from build123d import *

# Parameters (mm, degrees)
SKETCH2_W           = 25.4
SKETCH2_H           = 25.4
BOSS_EXTRUDE1_DEPTH = 279.4
SKETCH4_W           = 19.05
SKETCH4_H           = 10.16
CUT_EXTRUDE1_DEPTH  = 280.9766776
SKETCH5_R           = 3.2639
CUT_EXTRUDE2_DEPTH  = 281.839473721
SKETCH6_R           = 3.2639
CUT_EXTRUDE3_DEPTH  = 281.839473721


with BuildPart() as part:
    # Sketch2 → Boss-Extrude1 (new body)
    with BuildSketch(Plane.XY):
        Rectangle(SKETCH2_W, SKETCH2_H)
    extrude(amount=BOSS_EXTRUDE1_DEPTH)

    # Sketch4 → Cut-Extrude1 (cut, through all)
    with BuildSketch(Plane.XY):
        Rectangle(SKETCH4_W, SKETCH4_H)
    extrude(amount=CUT_EXTRUDE1_DEPTH, mode=Mode.SUBTRACT)

    # Sketch5 → Cut-Extrude2 (cut, through all)
    with BuildSketch(Plane(origin=(0, 12.7, 0), x_dir=(1, 0, 0), z_dir=(0, 1, 0))):
        with Locations(Location((0, -15.24, 0), (0, 0, 270))):
            Circle(SKETCH5_R)
    extrude(amount=-CUT_EXTRUDE2_DEPTH, mode=Mode.SUBTRACT)

    # Sketch6 → Cut-Extrude3 (cut, through all)
    with BuildSketch(Plane(origin=(0, 12.7, 0), x_dir=(1, 0, 0), z_dir=(0, 1, 0))):
        with Locations(Location((0, -228.6, 0), (0, 0, 270))):
            Circle(SKETCH6_R)
    extrude(amount=-CUT_EXTRUDE3_DEPTH, mode=Mode.SUBTRACT)


solid = part.part
Source: CAD feature listing. Evaluate the final solid. Frame: model axes, mm. A direction names the side the tool comes from. Give positions to 0.01 mm unless a question says otherwise; leave off trailing zeros. Order: outer loops, then holes, each group sorted by start corner. A loop starts at its lowest first (then second) coordinate and runs counter-clockwise, first axis right, second up. Notation, with made-up numbers: (22.5, -24.5) -> (40.5, -24.5) arc R30 ccw to (40.5, 1.5) -> close; hole circle Ø2 at (53.5, -8.5). An arc over 180 degrees is marked (long way). Use a Markdown table: item, result.
1) Mould query, pull axis Y, two halves, no side actions, for faces 1 (the flat face through (-9.525, 0, 138)), 2 (the flat face through (0, -12.7, 138)), 3 (the cylindrical face through (-1.25, 8.943, 231.615)). Classes: +Y half, -Y half, draft (parallel to the pull), parting line (faces both ways), or undercut.
Answer list:
| item | result |
|---|---|
| face 1 | undercut |
| face 2 | -Y half |
| face 3 | draft |
2) Section query D-D, the plane z = 62.5. Return the cut outline in (x, y) (3 decimals), then the cut area to 3 significant figures.
Answer list:
| item | result |
|---|---|
| outline | (-12.7, -12.7) -> (12.7, -12.7) -> (12.7, 12.7) -> (-12.7, 12.7) -> close; hole (-9.525, -5.08) -> (9.525, -5.08) -> (9.525, 5.08) -> (-9.525, 5.08) -> close |
| area | 452 mm² |
3) Ray query, line 1 along Y through (x, z) = (-5.25, 156); line 2 along X through (y, z) = (9, 15.24); line 3 along X through (y, z) = (-0.5, 154) (3 decimals). Return the intervals inside material, ascending. Write a range as [from, to].
Answer list:
| item | result |
|---|---|
| line 1 | [-12.7, -5.08], [5.08, 12.7] |
| line 2 | [-12.7, -3.26], [3.26, 12.7] |
| line 3 | [-12.7, -9.525], [9.525, 12.7] |
4) Section query C-C, the plane x = 0. Return the cut outline in (y, z).
Answer list:
| item | result |
|---|---|
| outline | (-12.7, 0) -> (-5.08, 0) -> (-5.08, 11.98) -> (-12.7, 11.98) -> close; (-12.7, 18.5) -> (-5.08, 18.5) -> (-5.08, 225.34) -> (-12.7, 225.34) -> close; (-12.7, 231.86) -> (-5.08, 231.86) -> (-5.08, 279.4) -> (-12.7, 279.4) -> close; (5.08, 0) -> (12.7, 0) -> (12.7, 11.98) -> (5.08, 11.98) -> close; (5.08, 18.5) -> (12.7, 18.5) -> (12.7, 225.34) -> (5.08, 225.34) -> close; (5.08, 231.86) -> (12.7, 231.86) -> (12.7, 279.4) -> (5.08, 279.4) -> close |
5) Section query B-B, the plane z = 228.6. Return the cut outline in (x, y) (3 decimals), then the cut area to 3 significant figures.
Answer list:
| item | result |
|---|---|
| outline | (-12.7, -12.7) -> (-3.264, -12.7) -> (-3.264, -5.08) -> (-9.525, -5.08) -> (-9.525, 5.08) -> (-3.264, 5.08) -> (-3.264, 12.7) -> (-12.7, 12.7) -> close; (3.264, -12.7) -> (12.7, -12.7) -> (12.7, 12.7) -> (3.264, 12.7) -> (3.264, 5.08) -> (9.525, 5.08) -> (9.525, -5.08) -> (3.264, -5.08) -> close |
| area | 352 mm² |
6) Section query A-A, the plane y = -2.25. Return the cut outline in (x, z) (3 decimals).
Answer list:
| item | result |
|---|---|
| outline | (-12.7, 0) -> (-9.525, 0) -> (-9.525, 279.4) -> (-12.7, 279.4) -> close; (9.525, 0) -> (12.7, 0) -> (12.7, 279.4) -> (9.525, 279.4) -> close |
7) Reachability of faces 4 (the flat face through (0, 12.7, 138)), 5 (the flat face through (0, -5.08, 138)) from +Z, -Z, +X, -X, +Y, -Y: full face, straight path, thin tool, end or side. Return the list, or none.
Answer list:
| item | result |
|---|---|
| face 4 | +Z, -Z, +X, -X, +Y |
| face 5 | +Z, -Z |
